The listing builds one solid part. Answer for the finished solid, in the listing's coordinates (mm). A direction names the side the tool comes from. Round coordinates to 2 decimals unless told otherwise and drop trailing zeros. Write each loop counter-clockwise with the first axis right and the second up, starting at its lowest first coordinate (ties: lowest second). Pieces come first, ordered by that corner, then holes. Notation, with made-up numbers: M 17.25,62.25 L 32.25,62.25 A23 ccw 32.25,73.25 Z; hole C 87.25,2 d10. An arc over 180 degrees is marked long. One line per item, written item: value. Start each with the question number.
(1) For a pull along Z with two mould halves and no side action, classify faces 4 (the flat face through (22, -2, -8)), 5 (the flat face through (54, -2, 0)), 6 (the flat face through (-56.5, -2, -12)), 7 (the flat face through (1, -2, 15)) as released by +Z, released by -Z, zero draft, split by the parting line, or undercut.
(2) Consider probe 1 along X at (y, z) = (-1.2, -7.25); probe 2 along Z at (x, y) = (-30, -1.55); probe 3 along X at (y, z) = (-0.4, -4). Determine where each line is inside the solid, lowest interval first.
(3) Given P1, Ø2, axis at y = -1.5, z = -5, coming from the -X side; P2, Ø2, axis at y = -3, z = -5, coming from the +X side, each flat-ended and moving along its own axis, determine where each tip first touches the part or whether it passes through.
(4) Section B-B (y = -3.2) is taken. Determine the outline of the cut face in (x, z), plus the area to 3 significant figures.
(5) For faces 1 (the flat face through (52.5, -2, -5)), 2 (the flat face through (32, -2, -10)), 3 (the flat face through (-54, -2, -10)), determine the directions among +Z, -Z, +X, -X, +Y, -Y from which every point of the face is accessible in a straight line to the end or side of a thin tool.
(6) Section A-A (x = 38) is taken. Determine the outline of the cut face in (y, z), plus the area to 3 significant figures.
(7) Section C-C (z = -7.5) is taken. Determine the outline of the cut face in (x, y), plus the area to 3 significant figures.
```python
from build123d import *

# Parameters (mm, degrees)
F0_W     = 20
F0_H     = 4
F1_DEPTH = 4


with BuildPart() as f1:
    # F0 (on Front) → F1 (new body)
    with BuildSketch(Plane.XZ):
        Polygon((56.5, 0), (56.5, 15), (-56.5, 15), (-56.5, 0), (-52.5, 0), (-52.5, -10), (-56.5, -10), (-56.5, -15), (56.5, -15), (56.5, -10), (52.5, -10), (52.5, 0), align=None)
        with Locations((-32, -8)):
            Rectangle(F0_W, F0_H, mode=Mode.SUBTRACT)
        with Locations((32, -8)):
            Rectangle(F0_W, F0_H, mode=Mode.SUBTRACT)
    extrude(amount=F1_DEPTH)


solid = f1.part
```
Recorded:
1. face 4: undercut
1. face 5: undercut
1. face 6: zero draft
1. face 7: released by +Z
2. probe 1: x = -52.5 to -42, -22 to 22, 42 to 52.5
2. probe 2: z = -15 to -10, -6 to 15
2. probe 3: x = -52.5 to 52.5
3. P1: stops at x = -52.5
3. P2: stops at x = 52.5
4. outline: M -56.5,-15 L 56.5,-15 L 56.5,-10 L 52.5,-10 L 52.5,0 L 56.5,0 L 56.5,15 L -56.5,15 L -56.5,0 L -52.5,0 L -52.5,-10 L -56.5,-10 Z; hole M -42,-10 L -22,-10 L -22,-6 L -42,-6 Z; hole M 22,-10 L 42,-10 L 42,-6 L 22,-6 Z
4. area: 3,150 mm2
5. face 1: +X, +Y, -Y
5. face 2: +Y, -Y
5. face 3: -X, +Y, -Y
6. outline: M -4,-15 L 0,-15 L 0,-10 L -4,-10 Z; M -4,-6 L 0,-6 L 0,15 L -4,15 Z
6. area: 104 mm2
7. outline: M -52.5,-4 L -42,-4 L -42,0 L -52.5,0 Z; M -22,-4 L 22,-4 L 22,0 L -22,0 Z; M 42,-4 L 52.5,-4 L 52.5,0 L 42,0 Z
7. area: 260 mm2
